Autodesk Inventor part; units mm, degrees
ref_plane "YZ Plane" through (0, 0, 0) normal (1, 0, 0) x (0, 1, 0)
ref_plane "XZ Plane" through (0, 0, 0) normal (0, 1, 0) x (-1, 0, 0)
ref_plane "XY Plane" through (0, 0, 0) normal (0, 0, 1) x (1, 0, 0)
sketch "Sketch1" plane through (0, 0, 0) normal (0, 1, 0) x (-1, 0, 0)
  line L0 (-36.5, 50) -> (-36.5, 45)
  circle A0 centre (45, 45) radius 1.5
  circle A1 centre (-45, -45) radius 1.5
  circle A2 centre (45, -45) radius 1.5
  circle A3 centre (-45, 45) radius 1.5
  line L1 (-50, 50) -> (50, 50)
  line L2 (-50, -50) -> (-50, 50)
  line L3 (50, -50) -> (-50, -50)
  line L4 (50, 50) -> (50, -50)
  line L5 (40, 45) -> (-40, 45)
  line L6 (40, 40) -> (40, 45)
  line L7 (45, 40) -> (40, 40)
  line L8 (45, -40) -> (45, 40)
  line L9 (40, -40) -> (45, -40)
  line L10 (40, -45) -> (40, -40)
  line L11 (-40, -45) -> (40, -45)
  line L12 (-40, -40) -> (-40, -45)
  line L13 (-45, -40) -> (-40, -40)
  line L14 (-45, 40) -> (-45, -40)
  line L15 (-40, 40) -> (-45, 40)
  line L16 (-40, 45) -> (-40, 40)
  line L17 (50, 50) -> (40, 50)
  line L18 (40, 50) -> (40, -50)
  line L19 (40, -50) -> (50, -50)
  line L20 (50, -50) -> (50, 50)
  line L21 (-82.5, 82.5) -> (-82.5, -82.5)
  line L22 (80, 17.5) -> (40, 17.5)
  line L23 (40, 17.5) -> (40, -17.5)
  line L24 (40, -17.5) -> (80, -17.5)
  line L25 (80, -17.5) -> (80, 17.5)
  point P0 (0, 0)
  point P1 (0, 0)
  point P2 (0, 0)
  point P3 (40, 0)
  point P4 (80, 0)
  dimension "d3" = 35
  dimension "d19" = 40
extrude "Extrusion1" add sketch "Sketch1" along normal blind 6 contours L1 L4 L22 L8 L7 L6 L18 | L7 L8 L22 L18 | L18 L10 L9 L8 L24 L4 L3 | L22 L25 L24 L4 | L4 L24 L8 L22 | L22 L8 L24 L18 | L24 L8 L9 L18
pattern_circular "Circular Pattern1" count 4 over 360 about axis through (0, -10, 0) along (0, 1, 0) of "Extrusion1"
sketch "Sketch2" plane through (80, 0, 17.5) normal (1, 0, 0) x (0, 0, -1)
  line L0 (0, 0) -> (35, 0)
  line L1 (35, 0) -> (35, 6)
  line L2 (0, 6) -> (35, 6)
  line L3 (0, 0) -> (0, 6)
  line L4 (0, 6) -> (0, 0)
  line L5 (0, 3) -> (35, 3)
  line L6 (17.5, 3) -> (35, 3)
  line L7 (17.5, 3) -> (0, 3)
  point P0 (17.5, 0)
  point P1 (8.75, 3)
  point P2 (26.25, 3)
hole "Hole1" at (80, 3, 8.75) at (80, 3, -8.75) direction (-1, 0, 0) diameter 3 depth 10 tip angle 118
pattern_circular "Circular Pattern2" count 4 over 360 about axis through (0, -10, 0) along (0, 1, 0) of "Hole1"
sketch "Sketch3" plane through (0, 0, 0) normal (0, -1, 0) x (1, 0, 0)
  line L0 (-50, -50) -> (-40, -50)
  line L1 (-40, -50) -> (-40, -40)
  line L2 (-40, -40) -> (-50, -40)
  line L3 (-50, -40) -> (-50, -50)
  line L4 (50, -50) -> (40, -50)
  line L5 (40, -50) -> (40, -40)
  line L6 (40, -40) -> (50, -40)
  line L7 (50, -40) -> (50, -50)
  line L8 (50, 50) -> (40, 50)
  line L9 (40, 50) -> (40, 40)
  line L10 (40, 40) -> (50, 40)
  line L11 (50, 40) -> (50, 50)
  line L12 (-50, 50) -> (-17.5, 50)
  line L13 (-50, 50) -> (-40, 50)
  line L14 (-40, 50) -> (-40, 40)
  line L15 (-40, 40) -> (-50, 40)
  line L16 (-50, 40) -> (-50, 50)
  circle A0 centre (-45, 45) radius 1.5
  circle A1 centre (45, 45) radius 1.5
  circle A2 centre (-45, -45) radius 1.5
  circle A3 centre (45, -45) radius 1.5
  circle A4 centre (45, 45) radius 7.0711
  line L17 (-40, 40) -> (-40, -40)
  circle A5 centre (-45, 45) radius 7.0711
  circle A6 centre (-45, -45) radius 7.0711
  line L18 (50, -50) -> (17.5, -50)
  circle A7 centre (45, -45) radius 7.0711
  point P0 (0, 0)
  dimension "d20" = 10
  dimension "d21" = 10
  dimension "d22" = 10
  dimension "d23" = 10
  dimension "d24" = 10
  dimension "d25" = 10
  dimension "d26" = 10
  dimension "d27" = 10
extrude "Extrusion2" add sketch "Sketch3" along normal blind 5 and the other way blind 6
fillet "Fillet4" radius 3 8 edges at (-17.5, 3, 80) (-80, 3, 17.5) (-80, 3, -17.5) (-17.5, 3, -80) (17.5, 3, -80) (80, 3, -17.5) (80, 3, 17.5) (17.5, 3, 80)
extrude "Extrusion3" add sketch "Sketch3" along normal blind 10 contours L3 L2 L1 L0 | L15 L16 L12 L14 | L4 L5 L6 L7 | L11 L10 L9 L8
properties part number "solar roof" material "ABS Plastic"
Source: CAD feature listing. Evaluate the final solid. Frame: model axes, mm. A direction names the side the tool comes from. Coordinates: 2 decimals unless noted, no trailing zeros. Write each loop counter-clockwise with the first axis right and the second up, starting at its lowest first coordinate (ties: lowest second). Pieces come first, ordered by that corner, then holes. Notation, with made-up numbers: (-7, 56) - (44, 56) arc R19 ccw to (44, 86) - close; hole circle Ø10 at (-25, 77.25). An arc over 180 degrees is marked (long way). Answer as a JSON object with one key per item and string values.
Q1. Section query C-C, the plane x = 0. Output: boundary loops of the cut face in (y, z), plus the area to 3 significant figures.
Ans:
{"outline": "(0, -80) - (6, -80) - (6, -40) - (0, -40) - close; (0, 40) - (6, 40) - (6, 80) - (0, 80) - close", "area": "480 mm2"}
Q2. Section query D-D, the plane x = 57. Output: boundary loops of the cut face in (y, z), plus the area to 3 significant figures.
Ans:
{"outline": "(0, -17.5) - (6, -17.5) - (6, 17.5) - (0, 17.5) - close", "area": "210 mm2"}
Q3. Draft query along Z for faces 4 (the flat face through (0, 3, -80)), 5 (the flat face through (-45, -7, 40)), 6 (the flat face through (-40, -7, 45)), 7 (the cylindrical face through (48.801, -0.645, -50.962)). Return one class per face: released by +Z, released by -Z, zero draft, split by the parting line, or undercut.
Ans:
{"face 4": "released by -Z", "face 5": "undercut", "face 6": "zero draft", "face 7": "undercut"}
Q4. Section query A-A, the plane y = -7.5. Output: boundary loops of the cut face in (x, z), plus the area to 3 significant figures.
Ans:
{"outline": "(-50, -50) - (-40, -50) - (-40, -40) - (-50, -40) - close; (-50, 40) - (-40, 40) - (-40, 50) - (-50, 50) - close; (40, -50) - (50, -50) - (50, -40) - (40, -40) - close; (40, 40) - (50, 40) - (50, 50) - (40, 50) - close; hole circle Ø3 at (-45, -45); hole circle Ø3 at (-45, 45); hole circle Ø3 at (45, -45); hole circle Ø3 at (45, 45)", "area": "372 mm2"}
Q5. First-contact query: pin 1 Ø2.5 at (x, z) = (-38.5, 46.5) entering from -Y; pin 2 Ø5 at (x, y) = (23.5, 2.5) entering from +Z; pin 3 Ø1 at (x, z) = (-17, 60.5) entering from -Y. Flat tips, straight axial feed; report the tip coordinate or a pass-through.
Ans:
{"pin 1": "stops at y = -5", "pin 2": "stops at z = 50", "pin 3": "stops at y = 0"}
Q6. Material intervals for line 1 (Z direction, x = 45, y = -3.25); line 2 (Z direction, x = -75.25, y = 3), sorted ascending. Write a range as [from, to].
Ans:
{"line 1": "z = [-52.07, -46.5], [-43.5, -37.93], [37.93, 43.5], [46.5, 52.07]", "line 2": "z = [-17.5, -10.25], [-7.25, 7.25], [10.25, 17.5]"}
Q7. Section query B-B, the plane z = 32. Output: boundary loops of the cut face in (x, y).
Ans:
{"outline": "(-50, 0) - (-40, 0) - (-40, 6) - (-50, 6) - close; (40, 0) - (50, 0) - (50, 6) - (40, 6) - close"}
Q8. Set-up query: faces 1 (the flat face through (45, -7, 40)), 2 (the flat face through (-40, -7, -45)), 3 (the flat face through (45, -7, 50)). Return all of +Z, -Z, +X, -X, +Y, -Y with unobstructed straight access to the full face (end or side cutting, diameter ignored); none if empty.
Ans:
{"face 1": "+X, -X, -Y", "face 2": "+Z, -Z, -Y", "face 3": "+Z, +X, -X, -Y"}
